from build123d import *

# Parameters (mm, degrees)
F4_W      = 40
F4_H      = 10
F4_W_2    = 10
F4_H_2    = 4
F5_DEPTH  = 1.5
F6_DEPTH  = 20
F7_W      = 33
F7_H      = 4
F8_DEPTH  = 5
F9_SIZE2  = 2.99999
F9_SIZE   = 11.49999
F10_SIZE2 = 11.49999
F10_SIZE  = 2.99999
F11_W     = 1.5
F11_H     = 4
F12_DEPTH = 2


# Not quite as in the source:
# - a fillet or chamfer is up to 0.001 mm smaller than in the source, because OpenCascade refuses the exact size


with BuildPart() as f5:
    # F4 (on Top) → F5 (new body)
    with BuildSketch(Plane.XY):
        Rectangle(F4_W, F4_H)
        Rectangle(F4_W_2, F4_H_2, mode=Mode.SUBTRACT)
    extrude(amount=F5_DEPTH)

    # F4 (on Top) → F6 (join)
    with BuildSketch(Plane.XY):
        Rectangle(F4_W_2, F4_H_2)
    extrude(amount=F6_DEPTH)

    # F7 (on face) → F8 (join)
    with BuildSketch(Plane.XY.offset(20)):
        Rectangle(F7_W, F7_H)
    extrude(amount=-F8_DEPTH)

    # F9 (size 11.5 and 3 in the source; OpenCascade refuses exactly that, so slightly less here)
    f9_edges = [f5.edges().sort_by_distance(p)[0] for p in [
        (16.5, 0, 15),
    ]]
    f9_side = f5.faces().sort_by_distance((10.75, 0, 15))[0]
    chamfer(f9_edges, length=F9_SIZE, length2=F9_SIZE2, reference=f9_side)

    # F10 (size 3 and 11.5 in the source; OpenCascade refuses exactly that, so slightly less here)
    f10_edges = [f5.edges().sort_by_distance(p)[0] for p in [
        (-16.5, 0, 15),
    ]]
    f10_side = f5.faces().sort_by_distance((-16.5, 0, 17.5))[0]
    chamfer(f10_edges, length=F10_SIZE, length2=F10_SIZE2, reference=f10_side)

    # F11 (on face) → F12 (join)
    with BuildSketch(Plane.XY.offset(20)):
        with Locations((15.75, 0)):
            Rectangle(F11_W, F11_H)
        with Locations((-15.75, 0)):
            Rectangle(F11_W, F11_H)
    extrude(amount=F12_DEPTH)


solid = f5.part
Read the model definition and answer for the solid it produces. Units are mm, in the model's axes. A direction names the side the tool comes from. Round coordinates to 2 decimals unless told otherwise and drop trailing zeros. Loops run counter-clockwise (first coordinate to the right, second up) from the corner with the lowest first, then second, coordinate; pieces in that order, holes last.
Q1. Determine the mould class of faces 1 (the face through (0, 2, 12)), 2 (the face through (10.83, -0.03, 16.52)), 3 (the face through (0, 0, 0)), 4 (the face through (-5, 0, 8)) for opening direction Z: released by +Z, released by -Z, zero draft, split by the parting line, or undercut.
Q2. Which of the six approach directions +Z, -Z, +X, -X, +Y, -Y give full straight-line access (tool end or side, diameter ignored) to faces 5 (the face through (-10.67, -0.03, 16.48)), 6 (the face through (5, 0, 8)), 7 (the face through (0, 0, 20)), 8 (the face through (-16.5, 0, 20)), 9 (the face through (-0.3, 2.3, 1.5))?
Q3. Section B-B on x = 3 is taken. Write down the section's boundary in (y, z).
Q4. Section A-A on x = -10 is taken. Write down the section's boundary in (y, z), and give its area (3 significant figures).
Q5. Each of these flat-tipped pins is pushed along its axis until it touches: pin 1 (3 mm diameter, centred on y = 1, z = 19, fed in from -X); pin 2 (4.5 mm diameter, centred on y = -0.5, z = 9, fed in from -X); pin 3 (2 mm diameter, centred on y = 0.5, z = 20.5, fed in from +X). Where does it stop, or does it pass through?
Q6. Consider probe 1 along Y at (x, z) = (-3, 8.25); probe 2 along Z at (x, y) = (18, 2); probe 3 along Z at (x, y) = (-14.5, -1.25). Determine where each line is inside the solid, lowest interval first.
Q7. Section D-D on z = 18.5 is taken. Write down the section's boundary in (x, y), and give its area (3 significant figures).
Output:
1. face 1: zero draft
1. face 2: undercut
1. face 3: released by -Z
1. face 4: undercut
2. face 5: -X, +Y, -Y
2. face 6: +X, +Y, -Y
2. face 7: +Z, +Y, -Y
2. face 8: +Z, -X, +Y, -Y
2. face 9: none
3. outline: (-5, 0) - (5, 0) - (5, 1.5) - (2, 1.5) - (2, 20) - (-2, 20) - (-2, 1.5) - (-5, 1.5) - close
4. outline: (-5, 0) - (5, 0) - (5, 1.5) - (-5, 1.5) - close; (-2, 16.3) - (2, 16.3) - (2, 20) - (-2, 20) - close
4. area: 29.8 mm2
5. pin 1: stops at x = -16.5
5. pin 2: stops at x = -5
5. pin 3: stops at x = 16.5
6. probe 1: y = -2 to 2
6. probe 2: z = 0 to 1.5
6. probe 3: z = 0 to 1.5, 17.48 to 20
7. outline: (-16.5, -2) - (16.5, -2) - (16.5, 2) - (-16.5, 2) - close
7. area: 132 mm2
